Part model, mm, in its own coordinate system. Give positions to 0.01 mm unless a question says otherwise; leave off trailing zeros. Order: outer loops, then holes, each group sorted by start corner. A loop starts at its lowest first (then second) coordinate and runs counter-clockwise, first axis right, second up. Notation, with made-up numbers: M -23,16.5 L 21,16.5 A26 cw 21,54.5 Z; hole C 32.25,40.25 d6. An arc over 180 degrees is marked long. Return JSON: item names as keys, results as strings.
from build123d import *

# Parameters (mm, degrees)
PAD_DEPTH            = 1.8
SKETCH001_W          = 30
SKETCH001_H          = 10
POCKET_DEPTH         = 1.801
POCKET_DEPTH_BACK    = 0.001
FILLET_R             = 3
FILLET001_R          = 0.5
SKETCH002_W          = 5
SKETCH002_H          = 1.5
SKETCH002_W_2        = 50
SKETCH002_H_2        = 5
POCKET001_DEPTH      = 1.801
POCKET001_DEPTH_BACK = 0.001
FILLET002_R          = 2.49


with BuildPart() as part:
    # Sketch → Pad (new body)
    with BuildSketch(Plane.XY):
        Polygon((88, 0), (88, 60), (78.75, 60), (78.75, 64), (69.25, 64), (69.25, 60), (-73.25, 60), (-73.25, 64), (-82.75, 64), (-82.75, 60), (-88, 60), (-88, 0), (-82.75, 0), (-82.75, -4), (-73.25, -4), (-73.25, 0), (69.25, 0), (69.25, -4), (78.75, -4), (78.75, 0), align=None)
    extrude(amount=-PAD_DEPTH)

    # Sketch001 → Pocket (cut, two sides)
    with BuildSketch(Plane.XY) as pocket_sk:
        with Locations((0, 5)):
            Rectangle(SKETCH001_W, SKETCH001_H)
    extrude(amount=-POCKET_DEPTH, mode=Mode.SUBTRACT)
    extrude(pocket_sk.sketch, amount=POCKET_DEPTH_BACK, mode=Mode.SUBTRACT)

    # Fillet
    fillet_edges = [part.edges().sort_by_distance(p)[0] for p in [
        (88, 0, -0.9),
        (88, 60, -0.9),
        (-88, 60, -0.9),
        (-88, 0, -0.9),
        (15, 0, -0.9),
        (15, 10, -0.9),
        (-15, 10, -0.9),
        (-15, 0, -0.9),
    ]]
    fillet(fillet_edges, radius=FILLET_R)

    # Fillet001
    fillet001_edges = [part.edges().sort_by_distance(p)[0] for p in [
        (-82.75, -4, -0.9),
        (-73.25, -4, -0.9),
        (69.25, -4, -0.9),
        (78.75, -4, -0.9),
        (78.75, 64, -0.9),
        (69.25, 64, -0.9),
        (-73.25, 64, -0.9),
        (-82.75, 64, -0.9),
    ]]
    fillet(fillet001_edges, radius=FILLET001_R)

    # Sketch002 → Pocket001 (cut, two sides)
    with BuildSketch(Plane.XY) as pocket001_sk:
        with Locations((47.5, 54.25)):
            Rectangle(SKETCH002_W, SKETCH002_H)
        with Locations((47.5, 42.75)):
            Rectangle(SKETCH002_W, SKETCH002_H)
        with Locations((-77.5, 54.25)):
            Rectangle(SKETCH002_W, SKETCH002_H)
        with Locations((-77.5, 42.75)):
            Rectangle(SKETCH002_W, SKETCH002_H)
        with Locations((95, 44.5)):
            Rectangle(SKETCH002_W_2, SKETCH002_H_2)
    extrude(amount=-POCKET001_DEPTH, mode=Mode.SUBTRACT)
    extrude(pocket001_sk.sketch, amount=POCKET001_DEPTH_BACK, mode=Mode.SUBTRACT)

    # Fillet002
    fillet002_edges = [part.edges().sort_by_distance(p)[0] for p in [
        (70, 42, -0.9),
        (70, 47, -0.9),
        (88, 47, -0.9),
        (88, 42, -0.9),
    ]]
    fillet(fillet002_edges, radius=FILLET002_R)


solid = part.part
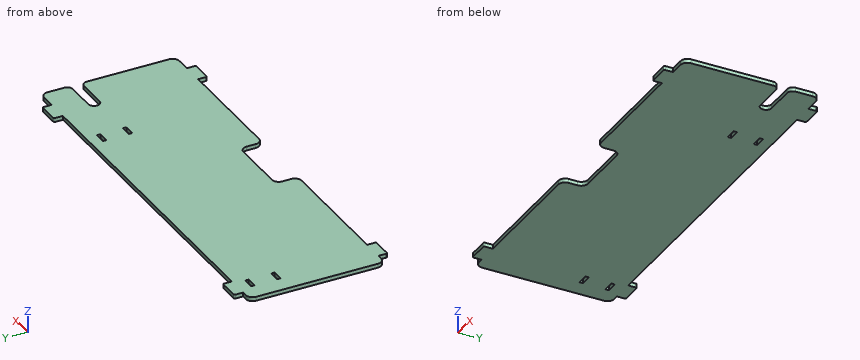
Q1. Band-saw the part on B-B (x = -31.5). Give the cut face in (y, z).
Established:
{"outline": "M 0,-1.8 L 60,-1.8 L 60,0 L 0,0 Z"}
Q2. Band-saw the part on A-A (z = -0.6). Give the number of separate pieces and of enclosed holes in the cut face, then the cut area to 3 significant figures.
Established:
{"separate pieces": "1", "enclosed holes": "4", "area": "10,300 mm²"}
Q3. Pin check, flat tips, straight feed: pin 1 (0.5 mm diameter, centred on x = 83, z = -1, fed in from -Y); pin 2 (0.5 mm diameter, centred on x = 10.5, z = -1, fed in from +Y). Stop position of each tip, or through.
Established:
{"pin 1": "stops at y = 0", "pin 2": "stops at y = 60"}
Q4. Probe line 1 along Y through (x, z) = (48, -0.1); line 2 along Y through (x, z) = (-77.5, -1.55); line 3 along Y through (x, z) = (80, -0.6). List the from-to ranges inside material, lowest first.
Established:
{"line 1": "y = 0 to 42, 43.5 to 53.5, 55 to 60", "line 2": "y = -4 to 42, 43.5 to 53.5, 55 to 64", "line 3": "y = 0 to 42, 47 to 60"}
